Source: CAD feature listing. Evaluate the final solid. Frame: model axes, mm. Give positions to 0.01 mm unless a question says otherwise; leave off trailing zeros. Write each loop counter-clockwise with the first axis right and the second up, starting at its lowest first coordinate (ties: lowest second). Pieces come first, ordered by that corner, then holes.
```python
from build123d import *

# Parameters (mm, degrees)
ESQUISSE1_R             = 6
BASE_EXTRUSION_DEPTH    = 130
CHANFREIN1_SIZE         = 1.5
ESQUISSE4_R             = 3
ENL_V_MAT_EXTRU_1_DEPTH = 10
ESQUISSE6_R             = 1.5
ENL_V_MAT_EXTRU_2_DEPTH = 10


with BuildPart() as part:
    # Esquisse1 → Base-Extrusion (new body)
    with BuildSketch(Plane.XY):
        Circle(ESQUISSE1_R)
    extrude(amount=-BASE_EXTRUSION_DEPTH)

    # Chanfrein1
    chanfrein1_edges = [part.edges().sort_by_distance(p)[0] for p in [
        (-6, 0, 0),
        (-6, 0, -130),
    ]]
    chamfer(chanfrein1_edges, length=CHANFREIN1_SIZE)

    # Esquisse4 → Enlèv. mat.-Extru.1 (cut, symmetric)
    with BuildSketch(Plane(origin=(0, 0, 0), x_dir=(1, 0, 0), z_dir=(0, 1, 0))):
        with Locations(Location((0, 10, 0), (0, 0, 270))):
            Circle(ESQUISSE4_R)
    extrude(amount=ENL_V_MAT_EXTRU_1_DEPTH, both=True, mode=Mode.SUBTRACT)

    # Esquisse6 → Enlèv. mat.-Extru.2 (cut, symmetric)
    with BuildSketch(Plane(origin=(0, 0, 0), x_dir=(0, 0, -1), z_dir=(1, 0, 0))):
        with Locations((38.4, 0)):
            Circle(ESQUISSE6_R)
    extrude(amount=ENL_V_MAT_EXTRU_2_DEPTH, both=True, mode=Mode.SUBTRACT)


solid = part.part
```
1. Cut plane D-D, the plane z = -75. Return the cut outline in (x, y).
2. Cut plane C-C, the plane z = -38.4. Return the cut outline in (x, y).
3. Cut plane A-A, the plane y = 0. Return the cut outline in (x, z), then the cut area to 3 significant figures.
4. Contact query for flat-ended pins moving along their axis: P1, Ø1, axis at x = -4, y = 3.5, coming from the +Z side; P2, Ø5, axis at y = 2.5, z = -20, coming from the -X side; P3, Ø1, axis at x = 4.5, z = -68.5, coming from the -Y side; P4, Ø3, axis at y = 4, z = -27.5, coming from the -X side. Output: stop coordinate, or through.
5. Line query: L1, parallel to Z at x = 1.5, y = 0; L2, parallel to Z at x = 1.5, y = 1.25; L3, parallel to Z at x = 0, y = 3.75. Output: solid intervals per line, ascending.
6. Mould query, pull axis Z, two halves, no side actions, for faces 1 (the cylindrical face through (0.08, 0.45, -39.83)), 2 (the flat face through (0, 0, 0)), 3 (the flat face through (0, 0, -130)). Classes: +Z half, -Z half, draft (parallel to the pull), parting line (faces both ways), or undercut.
7. Cut plane B-B, the plane x = 0. Return the cut outline in (y, z), then the cut area to 3 significant figures.
Response values:
1. outline: circle Ø12 at (0, 0)
2. outline: (-5.81, -1.5) arc R6 ccw to (5.81, -1.5) - close; (-5.81, 1.5) - (5.81, 1.5) arc R6 ccw to start
3. outline: (-6, -128.5) - (-4.5, -130) - (4.5, -130) - (6, -128.5) - (6, -39.9) - (-6, -39.9) - close; (-6, -36.9) - (6, -36.9) - (6, -1.5) - (4.5, 0) - (-4.5, 0) - (-6, -1.5) - close; hole circle Ø6 at (0, -10)
3. area: 1,490 mm2
4. P1: stops at z = -0.32
4. P2: stops at x = -6
4. P3: stops at y = -4.47
4. P4: stops at x = -5.45
5. L1: z = -130 to -39.9, -36.9 to -12.6, -7.4 to 0
5. L2: z = -130 to -39.23, -37.57 to -12.6, -7.4 to 0
5. L3: z = -130 to -13, -7 to 0
6. face 1: undercut
6. face 2: +Z half
6. face 3: -Z half
7. outline: (-6, -128.5) - (-4.5, -130) - (4.5, -130) - (6, -128.5) - (6, -13) - (-6, -13) - close; (-6, -7) - (6, -7) - (6, -1.5) - (4.5, 0) - (-4.5, 0) - (-6, -1.5) - close; hole circle Ø3 at (0, -38.4)
7. area: 1,480 mm2
